from build123d import *

# Parameters (mm, degrees)
SKETCH1_W                                    = 25.4
SKETCH1_H                                    = 38.1
SKETCH1_R                                    = 8.255
SKETCH1_R_2                                  = 1.1303
BOSS_EXTRUDE_WITH_4_40_TAP_DRILL_HOLES_DEPTH = 15.875
CUT_EXTRUDE1_REACH                           = 37.498
SKETCH3_W                                    = 26.67
SKETCH3_H                                    = 27.94
FILLET1_R                                    = 2.54
SKETCH5_R                                    = 1.65
CLEARANCE_HOLES_FOR_M3_SCREW_DEPTH           = 44.184668865


with BuildPart() as part:
    # Sketch1 → Boss-Extrude with 4-40 Tap Drill Holes (new, symmetric)
    with BuildSketch(Plane.XY):
        Rectangle(SKETCH1_W, SKETCH1_H)
        Circle(SKETCH1_R, mode=Mode.SUBTRACT)
        with Locations((-9.1313, 9.1313)):
            Circle(SKETCH1_R_2, mode=Mode.SUBTRACT)
        with Locations((9.1313, 9.1313)):
            Circle(SKETCH1_R_2, mode=Mode.SUBTRACT)
        with Locations((-9.1313, -9.1313)):
            Circle(SKETCH1_R_2, mode=Mode.SUBTRACT)
        with Locations((9.1313, -9.1313)):
            Circle(SKETCH1_R_2, mode=Mode.SUBTRACT)
    extrude(amount=BOSS_EXTRUDE_WITH_4_40_TAP_DRILL_HOLES_DEPTH, both=True)

    # Sketch3 → Cut-Extrude1 (cut, up to next)
    with BuildSketch(Plane(origin=(12.7, 0, 0), x_dir=(0, 0, -1), z_dir=(1, 0, 0)), mode=Mode.PRIVATE) as cut_extrude1_sk1:
        with Locations((2.54, 0)):
            Rectangle(SKETCH3_W, SKETCH3_H)
    cut_extrude1_tool1 = extrude(cut_extrude1_sk1.sketch, amount=-CUT_EXTRUDE1_REACH, mode=Mode.PRIVATE) & part.part
    add(cut_extrude1_tool1.solids().sort_by_distance((12.7, 0, -2.54))[0], mode=Mode.SUBTRACT)

    # Fillet1
    fillet1_edges = [part.edges().sort_by_distance(p)[0] for p in [
        (0, -13.97, 10.795),
        (0, 13.97, 10.795),
    ]]
    fillet(fillet1_edges, radius=FILLET1_R)

    # Sketch5 → Clearance Holes for M3 Screw (cut, through all)
    with BuildSketch(Plane(origin=(0, 19.05, 0), x_dir=(1, 0, 0), z_dir=(0, 1, 0))):
        with Locations(Location((-7.62, 10.795, 0), (0, 0, 270))):
            Circle(SKETCH5_R)
        with Locations(Location((-7.62, -4.445, 0), (0, 0, 270))):
            Circle(SKETCH5_R)
        with Locations(Location((7.62, -4.445, 0), (0, 0, 270))):
            Circle(SKETCH5_R)
        with Locations(Location((7.62, 10.795, 0), (0, 0, 270))):
            Circle(SKETCH5_R)
    extrude(amount=-CLEARANCE_HOLES_FOR_M3_SCREW_DEPTH, mode=Mode.SUBTRACT)


solid = part.part
For this review, take the finished solid that the model builds, in its own axes (mm). A direction names the side the tool comes from. Give positions to 0.01 mm unless a question says otherwise; leave off trailing zeros. Order: outer loops, then holes, each group sorted by start corner. A loop starts at its lowest first (then second) coordinate and runs counter-clockwise, first axis right, second up. Notation, with made-up numbers: M -9,68 L 22,68 A17 ccw 22,97 Z; hole C 15.25,15.25 d3. An arc over 180 degrees is marked long. Answer in a Markdown table with one row per item. Add a question column.
(1) For pin 1 (11.5 mm diameter, centred on x = -2, y = 3.5, fed in from -Z) (3 decimals), flat-tipped, find the tip position at first contact; note if it passes through.
(2) For faces 1 (the face through (-8.25, 16.55, -9.27)), 2 (the face through (0, 13.97, -4)), list the 3-axis set-ups (+Z, -Z, +X, -X, +Y, -Y) from which the entire face can be reached by the end or side of a thin tool; tool diameter is ignored.
(3) Wall thickness on probe 1 along Y at (x, z) = (10.5, -6); probe 2 along Z at (x, y) = (7.25, -7.5) (3 decimals); probe 3 along Y at (x, z) = (7, 13.5): over which ranges is each line inside the solid? List them lowest first. Write a range as [from, to].
(4) Mouldability with a two-part tool opening along Y and no side actions: class faces 3 (the face through (0, -19.05, 0)), 4 (the face through (7.874, 2.48, 13.299)), 5 (the face through (12.7, 0, 11)) as +Y half, -Y half, draft (parallel to the pull), parting line (faces both ways), or undercut.
(5) Consider section A-A on y = 15. State the section outline as (x, z) points (3 decimals), and give its area (3 significant figures).
(6) Consider section C-C on z = -7.5. State the section outline as (x, y) points.
(7) Consider section D-D on x = 1.5. State the section outline as (y, z) points (3 decimals).
(8) Consider section B-B on y = 0. State the section outline as (x, z) points (3 decimals).
Evaluation:
| question | item | result |
|---|---|---|
| 1 | pin 1 | stops at z = 10.795 |
| 2 | face 1 | +Y, -Y |
| 2 | face 2 | -Z, +X, -X |
| 3 | probe 1 | y = [-19.05, -13.97], [13.97, 19.05] |
| 3 | probe 2 | z = [10.795, 15.875] |
| 3 | probe 3 | y = [-19.05, -4.38], [4.38, 19.05] |
| 4 | face 3 | -Y half |
| 4 | face 4 | undercut |
| 4 | face 5 | draft |
| 5 | outline | M -12.7,-15.875 L 12.7,-15.875 L 12.7,15.875 L -12.7,15.875 Z; hole C -7.62,-10.795 d3.3; hole C -7.62,4.445 d3.3; hole C 7.62,-10.795 d3.3; hole C 7.62,4.445 d3.3 |
| 5 | area | 772 mm^2 |
| 6 | outline | M -12.7,-19.05 L 12.7,-19.05 L 12.7,-13.97 L -12.7,-13.97 Z; M -12.7,13.97 L 12.7,13.97 L 12.7,19.05 L -12.7,19.05 Z |
| 7 | outline | M -19.05,-15.875 L -13.97,-15.875 L -13.97,8.255 A2.54 cw -11.43,10.795 L -8.118,10.795 L -8.118,15.875 L -19.05,15.875 Z; M 8.118,10.795 L 11.43,10.795 A2.54 cw 13.97,8.255 L 13.97,-15.875 L 19.05,-15.875 L 19.05,15.875 L 8.118,15.875 Z |
| 8 | outline | M -12.7,10.795 L -8.255,10.795 L -8.255,15.875 L -12.7,15.875 Z; M 8.255,10.795 L 12.7,10.795 L 12.7,15.875 L 8.255,15.875 Z |
